Check sheet for the modelled part. Datum: model origin and axes. Units: mm. Round coordinates to 2 decimals unless told otherwise and drop trailing zeros. Write each loop counter-clockwise with the first axis right and the second up, starting at its lowest first coordinate (ties: lowest second). Pieces come first, ordered by that corner, then holes. Notation, with made-up numbers: M 32,51.25 L 42,51.25 A20 ccw 42,55.25 Z; hole C 39,33.5 d6. An arc over 180 degrees is marked long. Answer in a Markdown table with one row per item.
```python
from build123d import *

# Parameters (mm, degrees)
SKETCH1_W           = 80
SKETCH1_H           = 128
BOSS_EXTRUDE1_DEPTH = 1
FILLET1_R           = 4
SKETCH2_R           = 2.55
CUT_EXTRUDE1_DEPTH  = 76.478473752


with BuildPart() as part:
    # Sketch1 → Boss-Extrude1 (new body)
    with BuildSketch(Plane.XY):
        Rectangle(SKETCH1_W, SKETCH1_H)
    extrude(amount=BOSS_EXTRUDE1_DEPTH)

    # Fillet1
    fillet1_edges = [part.edges().sort_by_distance(p)[0] for p in [
        (40, -64, 0.5),
        (-40, -64, 0.5),
        (-40, 64, 0.5),
        (40, 64, 0.5),
    ]]
    fillet(fillet1_edges, radius=FILLET1_R)

    # Sketch2 → Cut-Extrude1 (cut, through all)
    with BuildSketch(Plane(origin=(0, 0, 0), x_dir=(-1, 0, 0), z_dir=(0, 0, -1))):
        with Locations((-33, -52.75)):
            Circle(SKETCH2_R)
        with Locations((-33, 52.75)):
            Circle(SKETCH2_R)
        with Locations((33, 52.75)):
            Circle(SKETCH2_R)
        with Locations((33, -52.75)):
            Circle(SKETCH2_R)
    extrude(amount=-CUT_EXTRUDE1_DEPTH, mode=Mode.SUBTRACT)


solid = part.part
```
1. Scan lines: L1, parallel to Y at x = 33, z = 0.75; L2, parallel to X at y = -55, z = 0.3. Record each from-to range of solid material in increasing order.
Found:
| item | result |
|---|---|
| L1 | y = -64 to -55.3, -50.2 to 50.2, 55.3 to 64 |
| L2 | x = -40 to -34.2, -31.8 to 31.8, 34.2 to 40 |
2. Section check B-B, the plane y = 52.75. Record the cut outline in (x, z), and give its area (3 significant figures).
Found:
| item | result |
|---|---|
| outline | M -40,0 L -35.55,0 L -35.55,1 L -40,1 Z; M -30.45,0 L 30.45,0 L 30.45,1 L -30.45,1 Z; M 35.55,0 L 40,0 L 40,1 L 35.55,1 Z |
| area | 69.8 mm2 |
3. Draft check along X on faces 1 (the face through (38.859, 62.797, 0.507)), 2 (the face through (-1, 1, 1)), 3 (the face through (35.548, 52.862, 0.493)). Enter one of: +X half, -X half, draft (parallel to the pull), parting line (faces both ways), or undercut.
Found:
| item | result |
|---|---|
| face 1 | +X half |
| face 2 | draft |
| face 3 | undercut |
4. Section check A-A, the plane x = 33. Record the cut outline in (y, z), and give its area (3 significant figures).
Found:
| item | result |
|---|---|
| outline | M -64,0 L -55.3,0 L -55.3,1 L -64,1 Z; M -50.2,0 L 50.2,0 L 50.2,1 L -50.2,1 Z; M 55.3,0 L 64,0 L 64,1 L 55.3,1 Z |
| area | 118 mm2 |
5. Go/stop test with a flat-tipped pin: pin 1 (1 mm diameter, centred on x = 21.5, y = 5.5, fed in from -Z). Record where the tip stops, or that it passes through.
Found:
| item | result |
|---|---|
| pin 1 | stops at z = 0 |
